Autodesk Fusion 360 part; units mm, degrees
sketch "Sketch1" plane through (0, 0, 0) normal (0, 0, 1) x (1, 0, 0)
  circle A0 centre (0, 0) radius 5.25
  circle A1 centre (0, 0) radius 3.1
  circle A2 centre (0, 0) radius 1.75
  circle A3 centre (0, 0) radius 3.4
  dimension "d1" = 10.5
  dimension "d2" = 6.2
  dimension "d3" = 3.5
  dimension "d8" = 6.8
extrude "Extrude1" add sketch "Sketch1" along normal blind 9.5 contours A1
extrude "Extrude2" add sketch "Sketch1" along normal blind 2 contours A0 | A3
extrude "Extrude3" add sketch "Sketch1" along normal blind 4 and the other way blind -4.5 contours A3
chamfer "Chamfer1" distance 0.2 angle 45 2 edges at (-3.1699, -1.2295, 4) (-3.1699, -1.2295, 4.5)
chamfer "Chamfer2" distance 0.5 angle 45 1 edges at (-1.6316, 0.6328, 0)
Geometry check sheet. Reference: the model listing, model coordinates, mm. A direction names the side the tool comes from. Give positions to 0.01 mm unless a question says otherwise; leave off trailing zeros. Order: outer loops, then holes, each group sorted by start corner. A loop starts at its lowest first (then second) coordinate and runs counter-clockwise, first axis right, second up. Notation, with made-up numbers: (42, 25.25) - (79, 25.25) arc R34 ccw to (79, 63.25) - close; hole circle Ø3 at (33, 39). An arc over 180 degrees is marked (long way). Write item = value, one per line. Start each with the question number.
1) Gauge pin test, flat ends, axial feed: pin 1 Ø1.5 at (x, z) = (-1.5, 3) entering from -Y; pin 2 Ø1.5 at (x, y) = (-1, -2.5) entering from -Z; pin 3 Ø1.5 at (x, z) = (-2.5, 6.5) entering from +Y. Record the tip position at first contact, or that the pin passes through.
2) Access from +Z, -Z, +X, -X, +Y, -Y to the whole of each face (thin tool, end or side, straight path). Record for faces 1 (the cylindrical face through (1.43, 2.75, 6.96)), 2 (the cylindrical face through (5, -1.6, 1)).
3) Scan lines: L1, parallel to Y at x = 0, z = 7.5; L2, parallel to X at y = -4, z = 1.5; L3, parallel to Z at x = 4, y = 1.5. Record each from-to range of solid material in increasing order.
4) Draft check along Z on faces 3 (the flat face through (2, 0, 9.5)), 4 (the cylindrical face through (1.43, 2.75, 2.99)), 5 (the cylindrical face through (1.617, 0.67, 4.937)), 6 (the flat face through (2.3, -1.1, 0)). Enter one of: released by +Z, released by -Z, zero draft, split by the parting line, or undercut.
5) Section check D-D (x = 4.25). Enter the section's corners in (y, z), then the cut area to 3 significant figures.
6) Section check A-A (x = 0). Enter the section's corners in (y, z).
7) Section check C-C (z = 5.75). Enter the section's corners in (x, y).
Geometry check:
q1.pin_1 = -3.01
q1.pin_2 = 0
q1.pin_3 = 2.56
q2.face_1 = +Z
q2.face_2 = +Z, -Z
q3.L1 = -3.1 to -1.75, 1.75 to 3.1
q3.L2 = -3.4 to 3.4
q3.L3 = 0 to 2
q4.face_3 = released by +Z
q4.face_4 = undercut
q4.face_5 = zero draft
q4.face_6 = released by -Z
q5.outline = (-3.08, 0) - (3.08, 0) - (3.08, 2) - (-3.08, 2) - close
q5.area = 12.3 mm2
q6.outline = (-5.25, 0) - (-2.25, 0) - (-1.75, 0.5) - (-1.75, 9.5) - (-3.1, 9.5) - (-3.1, 4.5) - (-3.2, 4.5) - (-3.4, 4.3) - (-3.4, 4.2) - (-3.2, 4) - (-3.1, 4) - (-3.1, 2) - (-5.25, 2) - close; (1.75, 0.5) - (2.25, 0) - (5.25, 0) - (5.25, 2) - (3.1, 2) - (3.1, 4) - (3.2, 4) - (3.4, 4.2) - (3.4, 4.3) - (3.2, 4.5) - (3.1, 4.5) - (3.1, 9.5) - (1.75, 9.5) - close
q7.outline = circle Ø6.2 at (0, 0); hole circle Ø3.5 at (0, 0)
